For this review, take the finished solid that the model builds, in its own axes (mm). A direction names the side the tool comes from. Round coordinates to 2 decimals unless told otherwise and drop trailing zeros. Order: outer loops, then holes, each group sorted by start corner. A loop starts at its lowest first (then second) coordinate and runs counter-clockwise, first axis right, second up.
from build123d import *

# Parameters (mm, degrees)
SKETCH1_R                = 140
SKETCH1_R_2              = 97
BOSS_EXTRUDE1_DEPTH      = 225
SKETCH2_R                = 23.5
BOSS_EXTRUDE2_DEPTH      = 32
CUT_EXTRUDE3_REACH       = 481.493
CUT_EXTRUDE3_END_RADIUS  = 97
SKETCH8_R                = 28
BOSS_EXTRUDE4_DEPTH      = 20
BOSS_EXTRUDE4_DEPTH_BACK = 37
SKETCH9_R                = 100
SKETCH9_R_2              = 50
SKETCH10_R               = 12
CUT_EXTRUDE4_DEPTH       = 20
SKETCH10_2_R             = 12
BOSS_EXTRUDE5_DEPTH      = 5


with BuildPart() as part:
    # Sketch1 → Boss-Extrude1 (new body)
    with BuildSketch(Plane(origin=(0, 0, 0), x_dir=(1, 0, 0), z_dir=(0, 1, 0))):
        with Locations(Location((0, 0, 0), (0, 0, 270))):
            Circle(SKETCH1_R)
        with Locations(Location((0, 0, 0), (0, 0, 270))):
            Circle(SKETCH1_R_2, mode=Mode.SUBTRACT)
    extrude(amount=-BOSS_EXTRUDE1_DEPTH)

    # Sketch2 → Boss-Extrude2 (add)
    # profile 1 of 3: a face of its own
    with BuildSketch(Plane(origin=(0, 0, 0), x_dir=(1, 0, 0), z_dir=(0, 1, 0))):
        with BuildLine():
            Line((50, 180), (50, 140))
            ThreePointArc((50, 140), (46.560641243, 121.776205471), (36.715732519, 106.059537635))
            Line((36.715732519, 106.059537635), (-36.715732519, 106.059537635))
            ThreePointArc((-36.715732519, 106.059537635), (-46.560641243, 121.776205471), (-50, 140))
            Line((-50, 140), (-50, 180))
            ThreePointArc((-50, 180), (0, 230), (50, 180))
        make_face()
        with Locations(Location((0, 180, 0), (0, 0, 270))):
            Circle(SKETCH2_R, mode=Mode.SUBTRACT)
    # profile 2 of 3: a face of its own
    with BuildSketch(Plane(origin=(0, 0, 0), x_dir=(1, 0, 0), z_dir=(0, 1, 0))):
        with BuildLine():
            Line((110.208120165, -21.233011737), (73.492387646, -84.826525898))
            ThreePointArc((73.492387646, -84.826525898), (82.180966893, -101.210800869), (96.24355653, -113.301270189))
            Line((96.24355653, -113.301270189), (130.884572681, -133.301270189))
            ThreePointArc((130.884572681, -133.301270189), (199.18584287, -115), (180.884572681, -46.698729811))
            Line((180.884572681, -46.698729811), (146.24355653, -26.698729811))
            ThreePointArc((146.24355653, -26.698729811), (128.741608136, -20.565404603), (110.208120165, -21.233011737))
        make_face()
        with Locations(Location((155.884572681, -90, 0), (0, 0, 270))):
            Circle(SKETCH2_R, mode=Mode.SUBTRACT)
    # profile 3 of 3: a face of its own
    with BuildSketch(Plane(origin=(0, 0, 0), x_dir=(1, 0, 0), z_dir=(0, 1, 0))):
        with BuildLine():
            Line((-73.492387646, -84.826525898), (-110.208120165, -21.233011737))
            ThreePointArc((-110.208120165, -21.233011737), (-128.741608136, -20.565404603), (-146.24355653, -26.698729811))
            Line((-146.24355653, -26.698729811), (-180.884572681, -46.698729811))
            ThreePointArc((-180.884572681, -46.698729811), (-199.18584287, -115), (-130.884572681, -133.301270189))
            Line((-130.884572681, -133.301270189), (-96.24355653, -113.301270189))
            ThreePointArc((-96.24355653, -113.301270189), (-82.180966893, -101.210800869), (-73.492387646, -84.826525898))
        make_face()
        with Locations(Location((-155.884572681, -90, 0), (0, 0, 270))):
            Circle(SKETCH2_R, mode=Mode.SUBTRACT)
    boss_extrude2 = extrude(amount=-BOSS_EXTRUDE2_DEPTH)

    # Mirror1: Boss-Extrude2 across plane
    add(boss_extrude2.mirror(Plane(origin=(0, -112.5, 0), x_dir=(0, 0, 1), z_dir=(0, -1, 0))))

    # Cut-Extrude3: up to this cylinder (the profile starts outside it)
    cut_extrude3_end = Plane(origin=(0, -112.5, 0), z_dir=(0, 1, 0)) * Cylinder(CUT_EXTRUDE3_END_RADIUS, 1157.986, mode=Mode.PRIVATE)
    # Sketch8 → Cut-Extrude3 (cut, up to the surface)
    with BuildSketch(Plane.XY.offset(140), mode=Mode.PRIVATE) as cut_extrude3_sk1:
        with Locations((0, -112.5)):
            Circle(SKETCH8_R)
    cut_extrude3_tool1 = extrude(cut_extrude3_sk1.sketch, amount=-CUT_EXTRUDE3_REACH, mode=Mode.PRIVATE) - cut_extrude3_end
    add(cut_extrude3_tool1.solids().sort_by_distance((0, -112.5, 140))[0], mode=Mode.SUBTRACT)

    # Sketch9 → Boss-Extrude4 (add, two sides: drawn at the far end of the back side and taken through both)
    with BuildSketch(Plane.XY.offset(140).offset(-BOSS_EXTRUDE4_DEPTH_BACK)):
        with Locations((0, -112.5)):
            Circle(SKETCH9_R)
        with Locations((0, -112.5)):
            Circle(SKETCH9_R_2, mode=Mode.SUBTRACT)
    extrude(amount=BOSS_EXTRUDE4_DEPTH + BOSS_EXTRUDE4_DEPTH_BACK)

    # Sketch10 → Cut-Extrude4 (cut)
    with BuildSketch(Plane.XY.offset(140)):
        with Locations((0, -37.5)):
            Circle(SKETCH10_R)
        with Locations((64.951905284, -150)):
            Circle(SKETCH10_R)
        with Locations((-64.951905284, -150)):
            Circle(SKETCH10_R)
    extrude(amount=CUT_EXTRUDE4_DEPTH, mode=Mode.SUBTRACT)

    # Sketch10<2> → Boss-Extrude5 (add)
    with BuildSketch(Plane.XY.offset(140)):
        with Locations((0, -37.5)):
            Circle(SKETCH10_2_R)
        with Locations((64.951905284, -150)):
            Circle(SKETCH10_2_R)
        with Locations((-64.951905284, -150)):
            Circle(SKETCH10_2_R)
    extrude(amount=BOSS_EXTRUDE5_DEPTH)


solid = part.part
(1) Tool access review of faces 4 (the face through (-148.2, -32, 67.6)), 5 (the face through (95.38, -82.46, 137.43)), 6 (the face through (-50, -209, -160)), 7 (the face through (134, -193, 81)): name each direction out of +Z, -Z, +X, -X, +Y, -Y from which nothing blocks a thin tool from reaching the whole face with its end or side.
(2) Add section C-C on y = -201. Give the boundary of the cut face in (x, z).
(3) Clearance check with flat-ended pins moving along their axes: P1, Ø4, axis at x = 51.5, y = -106, coming from the -Z side; P2, Ø4, axis at x = 123, y = -34.5, coming from the +Z side; P3, Ø7, axis at x = 4.5, y = -41.5, coming from the +Z side; P4, Ø10, axis at x = -163.5, z = 103, coming from the +Y side (3 decimals). State where each tip first meets the part, or that it passes through.
(4) Wall thickness on L1, parallel to X at y = -212, z = -180; L2, parallel to Y at x = -31.5, z = -157; L3, parallel to Z at x = -8, y = -200: over which ranges is each line inside the solid? List them lowest first.
(5) Add section B-B on x = -168. Give the boundary of the cut face in (y, z).
(6) Add section A-A on z = 0. Give the boundary of the cut face in (x, y), plus the area to 4 significant figures.
(7) Draft analysis for pull direction Z (two halves, no side actions). For faces 1 (the face through (-163.32, -15.78, 36.56)), 2 (the face through (-132.585, -209.224, 86.941)), 3 (the face through (-50, -16, -160)), state which applies: pulls with the +Z half, pulls with the -Z half, needs draft (parallel to the pull), parting line crosses it, or undercut.
(8) Add section D-D on x = 0. Count the separate pieces of the cut face and the enclosed holes in it, plus the area to 3 significant figures.
Here are the results:
1. face 4: +Z, -X
1. face 5: +Z
1. face 6: -Z, -X, +Y, -Y
1. face 7: +Z, +X
2. outline: (-180.88, 46.7) - (-146.24, 26.7) arc R50 ccw to (-138.11, 22.93) arc R140 ccw to (-49.2, -131.07) arc R50 ccw to (-50, -140) - (-50, -180) arc R50 ccw to (50, -180) - (50, -140) arc R50 ccw to (49.2, -131.07) arc R140 ccw to (138.11, 22.93) arc R50 ccw to (146.24, 26.7) - (180.88, 46.7) arc R50 ccw to (130.88, 133.3) - (96.24, 113.3) arc R50 ccw to (88.91, 108.14) arc R140 ccw to (46.56, 132.03) - (46.56, 160) - (-46.56, 160) - (-46.56, 132.03) arc R140 ccw to (-88.91, 108.14) arc R50 ccw to (-96.24, 113.3) - (-130.88, 133.3) arc R50 ccw to start; hole circle Ø47 at (-155.88, 90); hole circle Ø194 at (0, 0); hole circle Ø47 at (0, -180); hole circle Ø47 at (155.88, 90)
3. P1: stops at z = -130.96
3. P2: stops at z = 70.42
3. P3: stops at z = 145
3. P4: passes through
4. L1: x = -50 to -23.5, 23.5 to 50
4. L2: y = -225 to -193, -32 to 0
4. L3: z = -229.36 to -202.1, -157.9 to -96.67, 96.67 to 160
5. outline: (-225, 39.26) - (-193, 39.26) - (-193, 69.86) - (-225, 69.86) - close; (-225, 110.14) - (-193, 110.14) - (-193, 138.51) - (-225, 138.51) - close; (-32, 39.26) - (0, 39.26) - (0, 69.86) - (-32, 69.86) - close; (-32, 110.14) - (0, 110.14) - (0, 138.51) - (-32, 138.51) - close
6. outline: (-140, -225) - (-97, -225) - (-97, 0) - (-140, 0) - close; (97, -225) - (140, -225) - (140, 0) - (97, 0) - close
6. area: 19,350 mm2
7. face 1: pulls with the -Z half
7. face 2: undercut
7. face 3: needs draft
8. separate pieces: 5
8. enclosed holes: 0
8. area: 21,300 mm2
